```python
from build123d import *

# Parameters (mm, degrees)
EXTRUDE_1_DEPTH          = 0.5
EXTRUDE_1_2_DEPTH        = 0.5
CUT_EXTRUDE_1_DEPTH      = 10
CUT_EXTRUDE_1_DEPTH_BACK = 10
SKETCH_2_W               = 2
SKETCH_2_H               = 9.01144146
EXTRUDE_2_DEPTH          = 0.5
SKETCH_4_W               = 1
SKETCH_4_H               = 2
EXTRUDE_3_DEPTH          = 0.8
EXTRUDE_4_DEPTH          = 0.5
SKETCH_6_W               = 0.5
SKETCH_6_H               = 2
EXTRUDE_5_DEPTH          = 100


with BuildPart() as part:
    # Sketch 1 → Extrude 1 (new body)
    with BuildSketch(Plane(origin=(0, 0, 0), x_dir=(1, 0, 0), z_dir=(0, 1, 0))):
        with BuildLine():
            Line((-9.5, 23.5), (9.5, 23.5))
            ThreePointArc((9.5, 23.5), (10.207106781, 23.207106781), (10.5, 22.5))
            Line((10.5, 22.5), (10.5, 3.5))
            ThreePointArc((10.5, 3.5), (10.207106781, 2.792893219), (9.5, 2.5))
            Line((9.5, 2.5), (-9.5, 2.5))
            ThreePointArc((-9.5, 2.5), (-10.207106781, 2.792893219), (-10.5, 3.5))
            Line((-10.5, 3.5), (-10.5, 13.058292323))
            ThreePointArc((-10.5, 13.058292323), (-10.792893219, 13.765399104), (-11.5, 14.058292323))
            Line((-11.5, 14.058292323), (-25, 14.058292323))
            Line((-25, 14.058292323), (-25, 12.058292323))
            Line((-25, 12.058292323), (-13.5, 12.058292323))
            ThreePointArc((-13.5, 12.058292323), (-12.792893219, 11.765399104), (-12.5, 11.058292323))
            Line((-12.5, 11.058292323), (-12.5, 1.5))
            ThreePointArc((-12.5, 1.5), (-12.207106781, 0.792893219), (-11.5, 0.5))
            Line((-11.5, 0.5), (11.5, 0.5))
            ThreePointArc((11.5, 0.5), (12.207106781, 0.792893219), (12.5, 1.5))
            Line((12.5, 1.5), (12.5, 24.5))
            ThreePointArc((12.5, 24.5), (12.207106781, 25.207106781), (11.5, 25.5))
            Line((11.5, 25.5), (-11.5, 25.5))
            ThreePointArc((-11.5, 25.5), (-12.207106781, 25.207106781), (-12.5, 24.5))
            Line((-12.5, 24.5), (-12.5, 18.246362536))
            ThreePointArc((-12.5, 18.246362536), (-12.792893219, 17.539255755), (-13.5, 17.246362536))
            Line((-13.5, 17.246362536), (-25, 17.246362536))
            Line((-25, 17.246362536), (-25, 15.246362536))
            Line((-25, 15.246362536), (-11.5, 15.246362536))
            ThreePointArc((-11.5, 15.246362536), (-10.792893219, 15.539255755), (-10.5, 16.246362536))
            Line((-10.5, 16.246362536), (-10.5, 22.5))
            ThreePointArc((-10.5, 22.5), (-10.207106781, 23.207106781), (-9.5, 23.5))
        make_face()
    extrude(amount=EXTRUDE_1_DEPTH)


with BuildPart() as body_2:
    # Sketch 1 → Extrude 1 2 (new body)
    with BuildSketch(Plane(origin=(0, 0, 0), x_dir=(1, 0, 0), z_dir=(0, 1, 0))):
        with BuildLine():
            Line((-11.5, -0.5), (11.5, -0.5))
            ThreePointArc((11.5, -0.5), (12.207106781, -0.792893219), (12.5, -1.5))
            Line((12.5, -1.5), (12.5, -24.5))
            ThreePointArc((12.5, -24.5), (12.207106781, -25.207106781), (11.5, -25.5))
            Line((11.5, -25.5), (-11.5, -25.5))
            ThreePointArc((-11.5, -25.5), (-12.207106781, -25.207106781), (-12.5, -24.5))
            Line((-12.5, -24.5), (-12.5, -1.5))
            ThreePointArc((-12.5, -1.5), (-12.207106781, -0.792893219), (-11.5, -0.5))
        make_face()
        with BuildLine():
            Line((-9.5, -2.5), (9.5, -2.5))
            ThreePointArc((9.5, -2.5), (10.207106781, -2.792893219), (10.5, -3.5))
            Line((10.5, -3.5), (10.5, -22.5))
            ThreePointArc((10.5, -22.5), (10.207106781, -23.207106781), (9.5, -23.5))
            Line((9.5, -23.5), (-9.5, -23.5))
            ThreePointArc((-9.5, -23.5), (-10.207106781, -23.207106781), (-10.5, -22.5))
            Line((-10.5, -22.5), (-10.5, -3.5))
            ThreePointArc((-10.5, -3.5), (-10.207106781, -2.792893219), (-9.5, -2.5))
        make_face(mode=Mode.SUBTRACT)
    extrude(amount=EXTRUDE_1_2_DEPTH)


with BuildPart() as cut_extrude_1_tool:
    # Sketch 2 → Cut-Extrude 1 (new, two sides: drawn at the far end of the back side and taken through both)
    with BuildSketch(Plane(origin=(0, 0, 0), x_dir=(1, 0, 0), z_dir=(0, 1, 0)).offset(-CUT_EXTRUDE_1_DEPTH_BACK)):
        Rectangle(SKETCH_2_W, SKETCH_2_H)
    extrude(amount=CUT_EXTRUDE_1_DEPTH + CUT_EXTRUDE_1_DEPTH_BACK)


with BuildPart() as part_1:
    add(part.part)

    # Cut-Extrude 1: cut by cut_extrude_1_tool
    add(cut_extrude_1_tool.part, mode=Mode.SUBTRACT)



with BuildPart() as body_2_1:
    add(body_2.part)

    # Cut-Extrude 1: cut by cut_extrude_1_tool
    add(cut_extrude_1_tool.part, mode=Mode.SUBTRACT)


with BuildPart() as part_2:
    add(part_1.part)

    add(body_2_1.part)  # Extrude 2 merges body 2
    # Sketch 3 → Extrude 2 (add)
    with BuildSketch(Plane(origin=(0, 0, 0), x_dir=(1, 0, 0), z_dir=(0, 1, 0))):
        with BuildLine():
            Line((-1, 2.5), (-0.28379779, 2.176260251))
            ThreePointArc((-0.28379779, 2.176260251), (0.144512655, 1.807294997), (0.304305253, 1.265029821))
            Line((0.304305253, 1.265029821), (0.304305253, 0.459864337))
            ThreePointArc((0.304305253, 0.459864337), (0.46409785, -0.082400839), (0.892408295, -0.451366093))
            Line((0.892408295, -0.451366093), (1, -0.5))
            Line((1, -0.5), (1, -2.5))
            Line((1, -2.5), (0.28379779, -2.176260251))
            ThreePointArc((0.28379779, -2.176260251), (-0.144512655, -1.807294997), (-0.304305253, -1.265029821))
            Line((-0.304305253, -1.265029821), (-0.304305253, -0.459864337))
            ThreePointArc((-0.304305253, -0.459864337), (-0.46409785, 0.082400839), (-0.892408295, 0.451366093))
            Line((-0.892408295, 0.451366093), (-1, 0.5))
            Line((-1, 0.5), (-1, 2.5))
        make_face()
    extrude(amount=EXTRUDE_2_DEPTH)

    # Sketch 4 → Extrude 3 (add)
    with BuildSketch(Plane(origin=(0, 0, 0), x_dir=(1, 0, 0), z_dir=(0, 1, 0))):
        with Locations((-1.5, -1.5)):
            Rectangle(SKETCH_4_W, SKETCH_4_H)
        with Locations((1.5, 1.5)):
            Rectangle(SKETCH_4_W, SKETCH_4_H)
    extrude(amount=-EXTRUDE_3_DEPTH)

    # Sketch 5 → Extrude 4 (add)
    with BuildSketch(Plane(origin=(0, -0.8, 0), x_dir=(1, 0, 0), z_dir=(0, 1, 0))):
        with BuildLine():
            Line((-1, -2.5), (0.08384733, -1.594586619))
            ThreePointArc((0.08384733, -1.594586619), (0.348584902, -1.250746207), (0.442741007, -0.827134547))
            Line((0.442741007, -0.827134547), (0.442741007, -0.433160476))
            ThreePointArc((0.442741007, -0.433160476), (0.536897113, -0.009548815), (0.801634685, 0.334291597))
            Line((0.801634685, 0.334291597), (1, 0.5))
            Line((1, 0.5), (1, 2.5))
            Line((1, 2.5), (-0.08384733, 1.594586619))
            ThreePointArc((-0.08384733, 1.594586619), (-0.348584902, 1.250746207), (-0.442741007, 0.827134547))
            Line((-0.442741007, 0.827134547), (-0.442741007, 0.433160476))
            ThreePointArc((-0.442741007, 0.433160476), (-0.536897113, 0.009548815), (-0.801634685, -0.334291597))
            Line((-0.801634685, -0.334291597), (-1, -0.5))
            Line((-1, -0.5), (-1, -2.5))
        make_face()
    extrude(amount=EXTRUDE_4_DEPTH)

    # Sketch 6 → Extrude 5 (add)
    with BuildSketch(Plane(origin=(0, 0, 0), x_dir=(1, 0, 0), z_dir=(0, 1, 0))):
        with Locations((-24.75, 16.246362536)):
            Rectangle(SKETCH_6_W, SKETCH_6_H)
        with Locations((-24.75, 13.058292323)):
            Rectangle(SKETCH_6_W, SKETCH_6_H)
    extrude(amount=EXTRUDE_5_DEPTH)


solid = part_2.part
```
Could you check a few things on this model? Use its own coordinates, in mm. A direction names the side the tool comes from. Round coordinates to 2 decimals unless told otherwise and drop trailing zeros. Write each loop counter-clockwise with the first axis right and the second up, starting at its lowest first coordinate (ties: lowest second). Pieces come first, ordered by that corner, then holes.
(1) Which directions (+Z, -Z, +X, -X, +Y, -Y) give clear straight access to the entire face, cutting with the end or side of a thin tool? Please do faces 1 (the face through (0, -0.8, 0)), 2 (the face through (-24.5, 50, -16)).
Findings below:
face 1: +Z, -Z, +X, -X, -Y
face 2: +Z, -Z, +X, +Y
(2) Suppose I cut it at A-A on y = 63.5. Write out the boundary of the cut face in (x, z), and give its area (3 significant figures).
Findings below:
outline: (-25, -17.25) - (-24.5, -17.25) - (-24.5, -15.25) - (-25, -15.25) - close; (-25, -14.06) - (-24.5, -14.06) - (-24.5, -12.06) - (-25, -12.06) - close
area: 2.00 mm2
(3) Thinking about a two-plate mould opening in Y: for faces 3 (the face through (0, -0.3, 0)), 4 (the face through (-1, 0.5, -24)), 5 (the face through (-24.8, 49.8, -12.058)), which applies, +Y half, -Y half, draft (parallel to the pull), parting line (faces both ways), or undercut?
Findings below:
face 3: undercut
face 4: +Y half
face 5: draft
(4) Suppose I cut it at B-B on x = -5. Write out the boundary of the cut face in (y, z), and give its area (3 significant figures).
Findings below:
outline: (0, -25.5) - (0.5, -25.5) - (0.5, -23.5) - (0, -23.5) - close; (0, -2.5) - (0.5, -2.5) - (0.5, -0.5) - (0, -0.5) - close; (0, 0.5) - (0.5, 0.5) - (0.5, 2.5) - (0, 2.5) - close; (0, 23.5) - (0.5, 23.5) - (0.5, 25.5) - (0, 25.5) - close
area: 4.00 mm2
(5) If I drill on probe 1 along X at (y, z) = (17, -13), over which ranges is the centre line in solid material (lowest first)?
Findings below:
probe 1: x = -25 to -24.5
(6) Suppose I cut it at C-C on z = -6. Write out the boundary of the cut face in (x, y), and give its area (3 significant figures).
Findings below:
outline: (-12.5, 0) - (-10.5, 0) - (-10.5, 0.5) - (-12.5, 0.5) - close; (10.5, 0) - (12.5, 0) - (12.5, 0.5) - (10.5, 0.5) - close
area: 2.00 mm2
(7) For pin 1 (12 mm diameter, centred on x = -17.5, z = 7, fed in from -Y); pin 2 (11 mm diameter, centred on x = -12, z = 0.5, fed in from +Y), each with a flat end and sliding along its axis, tell me the tip position at first contact or that it passes through.
Findings below:
pin 1: stops at y = 0
pin 2: stops at y = 0.5
